Check sheet for the modelled part. Datum: model origin and axes. Units: mm. A direction names the side the tool comes from. Give positions to 0.01 mm unless a question says otherwise; leave off trailing zeros. Order: outer loops, then holes, each group sorted by start corner. A loop starts at its lowest first (then second) coordinate and runs counter-clockwise, first axis right, second up.
from build123d import *

# Parameters (mm, degrees)
F0_W     = 960
F0_H     = 350
F1_DEPTH = 144
F2_W     = 920
F2_H     = 310
F3_DEPTH = 124
F5_DEPTH = 20


with BuildPart() as f1:
    # F0 (on Top) → F1 (new body)
    with BuildSketch(Plane.XY):
        Rectangle(F0_W, F0_H)
    extrude(amount=F1_DEPTH)

    # F2 (on face) → F3 (cut)
    with BuildSketch(Plane.XY.offset(144)):
        Rectangle(F2_W, F2_H)
    extrude(amount=-F3_DEPTH, mode=Mode.SUBTRACT)

    # F4 (on face) → F5 (cut)
    with BuildSketch(Plane.XZ.offset(175)):
        with BuildLine():
            Line((125, 144), (-125, 144))
            add(Edge.make_bspline(
                [(-125, 144), (-75, 144), (-93.0105845008, 124.1732701609), (-37.6218932166, 91.8329972806), (37.6218932166, 91.8329972806), (93.0105845008, 124.1732701609), (75, 144), (125, 144)],
                knots=[0, 0, 0, 0, 0.1911314136, 0.3781938731, 0.6218061269, 0.8088685864, 1, 1, 1, 1], degree=3))
        make_face()
    extrude(amount=-F5_DEPTH, mode=Mode.SUBTRACT)


solid = f1.part
1) Material ranges on L1, parallel to X at y = 144, z = 22; L2, parallel to Y at x = 155, z = 89; L3, parallel to Z at x = 291.5, y = 60.5, recorded low to high.
Recorded:
L1: x = -480 to -460, 460 to 480
L2: y = -175 to -155, 155 to 175
L3: z = 0 to 20
2) Set-up check for faces 4 (the face through (480, -2, 71)), 5 (the face through (-6, 2, 20)): record each of +Z, -Z, +X, -X, +Y, -Y from which the full face is reachable in a straight line by a thin tool's end or side.
Recorded:
face 4: +Z, -Z, +X, +Y, -Y
face 5: +Z
3) Section check A-A, the plane z = 83. Record the cut outline in (x, y).
Recorded:
outline: (-480, -175) - (480, -175) - (480, 175) - (-480, 175) - close; hole (-460, -155) - (460, -155) - (460, 155) - (-460, 155) - close
4) Section check C-C, the plane y = -97. Record the cut outline in (x, z), then the cut area to 3 significant figures.
Recorded:
outline: (-480, 0) - (480, 0) - (480, 144) - (460, 144) - (460, 20) - (-460, 20) - (-460, 144) - (-480, 144) - close
area: 24,200 mm2
5) Depth check by flat-ended pin: pin 1 Ø12 at (x, y) = (278, 130.5) entering from +Z. Enter the tip coordinate at first touch or a pass-through.
Recorded:
pin 1: stops at z = 20
6) Draft check along Y on faces 1 (the face through (460, -2, 83)), 2 (the face through (-7, -175, 71)), 3 (the face through (-109, 156, 144)). Enter one of: +Y half, -Y half, draft (parallel to the pull), parting line (faces both ways), or undercut.
Recorded:
face 1: undercut
face 2: -Y half
face 3: draft
7) Section check B-B, the plane x = 158.5. Record the cut outline in (y, z).
Recorded:
outline: (-175, 0) - (175, 0) - (175, 144) - (155, 144) - (155, 20) - (-155, 20) - (-155, 144) - (-175, 144) - close
